Geometry check sheet. Reference: the model listing, model coordinates, mm. Face numbers are marked on the shaded views. Round coordinates to 2 decimals unless told otherwise and drop trailing zeros. Write each loop counter-clockwise with the first axis right and the second up, starting at its lowest first coordinate (ties: lowest second). Pieces come first, ordered by that corner, then holes. Notation, with made-up numbers: M 85,35 L 132,35 A15 ccw 132,59 Z; hole C 14.5,83 d9. An arc over 180 degrees is marked long. Put each result on its own line as item: value. Start each with the question number.
(1) Material ranges on probe 1 along Z at (x, y) = (-14.5, 1.5); probe 2 along X at (y, z) = (0.25, -1); probe 3 along Z at (x, y) = (-17, 0), recorded low to high.
(2) Gauge pin test, flat ends, axial feed: pin 1 (2 mm diameter, centred on y = 0, z = 1, fed in from +X); pin 2 (1 mm diameter, centred on x = -28, y = 1.5, fed in from -Z); pin 3 (1 mm diameter, centred on x = -5, y = -1.5, fed in from +Z). Record the tip position at first contact, or that the pin passes through.
(3) Mould release check, pull along Z, two halves, no side actions. Record for the marked faces 1, 2 and 3: pulls with the +Z half, pulls with the -Z half, needs draft (parallel to the pull), parting line crosses it, or undercut.
(4) Section check A-A on z = 0. Record the cut outline in (x, y), then the cut area to 3 significant figures.
(5) Section check B-B on x = -10.5. Record the cut outline in (y, z).
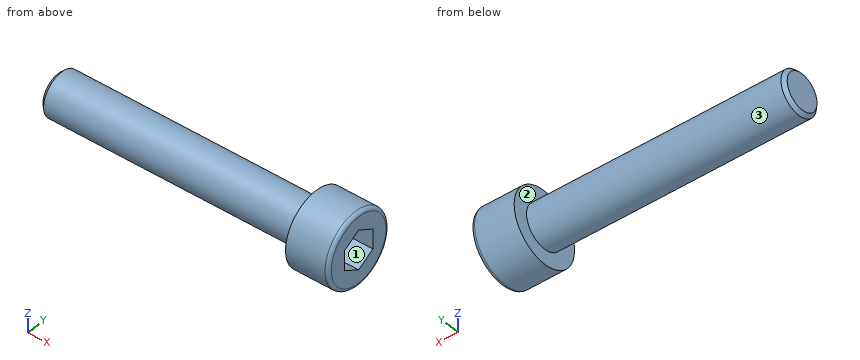
from build123d import *

# Parameters (mm, degrees)
SFAZOWANIE1_SIZE           = 0.4
ZAOKR_GLENIE1_R            = 0.4
WYTNIJ_WYCI_GNI_CIE1_DEPTH = 4


with BuildPart() as part:
    # Szkic1 → Obrót1 (revolve)
    with BuildSketch(Plane.XY):
        Polygon((0, 0), (0, 4.25), (-5, 4.25), (-5, 2.5), (-35, 2.5), (-35, 0), align=None)
    revolve(axis=Axis((-123.158940217, 0, 0), (1, 0, 0)))

    # Sfazowanie1
    sfazowanie1_edges = [part.edges().sort_by_distance(p)[0] for p in [
        (-35, -2.5, 0),
    ]]
    chamfer(sfazowanie1_edges, length=SFAZOWANIE1_SIZE)

    # Zaokrąglenie1
    zaokr_glenie1_edges = [part.edges().sort_by_distance(p)[0] for p in [
        (0, -4.25, 0),
    ]]
    fillet(zaokr_glenie1_edges, radius=ZAOKR_GLENIE1_R)

    # Szkic2 → Wytnij-wyciągnięcie1 (cut)
    with BuildSketch(Plane(origin=(0, 0, 0), x_dir=(0, 0, -1), z_dir=(1, 0, 0))):
        Polygon((2.309401077, 0), (1.154700538, 2), (-1.154700538, 2), (-2.309401077, 0), (-1.154700538, -2), (1.154700538, -2), align=None)
    extrude(amount=-WYTNIJ_WYCI_GNI_CIE1_DEPTH, mode=Mode.SUBTRACT)


solid = part.part
Answers follow:
1. probe 1: z = -2 to 2
1. probe 2: x = -35 to -4
1. probe 3: z = -2.5 to 2.5
2. pin 1: stops at x = -4
2. pin 2: stops at z = -2.29
2. pin 3: stops at z = 4.13
3. face 1: undercut
3. face 2: needs draft
3. face 3: parting line crosses it
4. outline: M -35,-2.1 L -34.6,-2.5 L -5,-2.5 L -5,-4.25 L -0.4,-4.25 A0.4 ccw 0,-3.85 L 0,-2 L -4,-2 L -4,2 L 0,2 L 0,3.85 A0.4 ccw -0.4,4.25 L -5,4.25 L -5,2.5 L -34.6,2.5 L -35,2.1 Z
4. area: 176 mm^2
5. outline: C 0,0 d5
